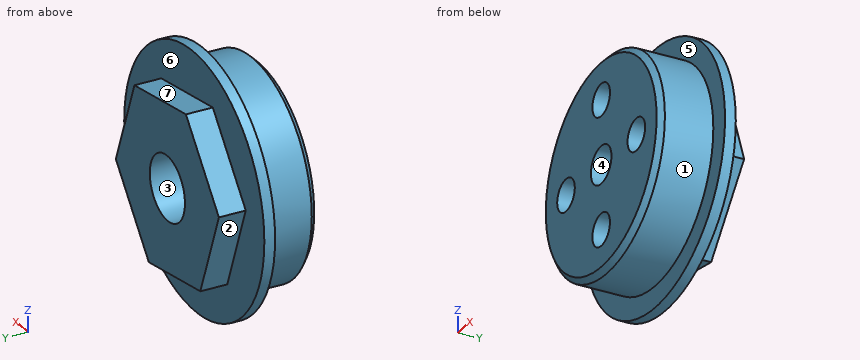
from build123d import *

# Parameters (mm, degrees)
ESQUISSE1_R             = 9.95
BOSS_EXTRU_1_DEPTH      = 6
BOSS_EXTRU_2_DEPTH      = 2.5
ESQUISSE3_R             = 11.95
ESQUISSE3_R_2           = 9.95
BOSS_EXTRU_3_DEPTH      = 1
ESQUISSE4_R             = 1.5
ENL_V_MAT_EXTRU_1_DEPTH = 5
ESQUISSE5_R             = 1.75
ENL_V_MAT_EXTRU_2_DEPTH = 9.5
ESQUISSE6_R             = 3
ENL_V_MAT_EXTRU_3_DEPTH = 3.5
CHANFREIN1_SIZE         = 0.5


with BuildPart() as part:
    # Esquisse1 → Boss.-Extru.1 (new body)
    with BuildSketch(Plane(origin=(0, 0, 0), x_dir=(1, 0, 0), z_dir=(0, 1, 0))):
        Circle(ESQUISSE1_R)
    extrude(amount=BOSS_EXTRU_1_DEPTH)

    # Esquisse2 → Boss.-Extru.2 (add)
    with BuildSketch(Plane(origin=(0, 6, 0), x_dir=(1, 0, 0), z_dir=(0, 1, 0))):
        Polygon((-3.162738548, -8.319079569), (5.623164969, -6.898551713), (8.785903517, 1.420527856), (3.162738548, 8.319079569), (-5.623164969, 6.898551713), (-8.785903517, -1.420527856), align=None)
    extrude(amount=BOSS_EXTRU_2_DEPTH)

    # Esquisse3 → Boss.-Extru.3 (add)
    with BuildSketch(Plane(origin=(0, 6, 0), x_dir=(1, 0, 0), z_dir=(0, 1, 0))):
        Circle(ESQUISSE3_R)
        Circle(ESQUISSE3_R_2, mode=Mode.SUBTRACT)
    extrude(amount=-BOSS_EXTRU_3_DEPTH)

    # Esquisse4 → Enlèv. mat.-Extru.1 (cut)
    with BuildSketch(Plane.XZ):
        with Locations((0, 6)):
            Circle(ESQUISSE4_R)
        with Locations((6, 0)):
            Circle(ESQUISSE4_R)
        with Locations((0, -6)):
            Circle(ESQUISSE4_R)
        with Locations((-6, 0)):
            Circle(ESQUISSE4_R)
    extrude(amount=-ENL_V_MAT_EXTRU_1_DEPTH, mode=Mode.SUBTRACT)

    # Esquisse5 → Enlèv. mat.-Extru.2 (cut, through all)
    with BuildSketch(Plane.XZ):
        Circle(ESQUISSE5_R)
    extrude(amount=-ENL_V_MAT_EXTRU_2_DEPTH, mode=Mode.SUBTRACT)

    # Esquisse6 → Enlèv. mat.-Extru.3 (cut)
    with BuildSketch(Plane(origin=(0, 8.5, 0), x_dir=(1, 0, 0), z_dir=(0, 1, 0))):
        Circle(ESQUISSE6_R)
    extrude(amount=-ENL_V_MAT_EXTRU_3_DEPTH, mode=Mode.SUBTRACT)

    # Chanfrein1
    chanfrein1_edges = [part.edges().sort_by_distance(p)[0] for p in [
        (-9.95, 0, 0),
    ]]
    chamfer(chanfrein1_edges, length=CHANFREIN1_SIZE)


solid = part.part
The model under review builds one solid part; all positions refer to its coordinate system, in mm. Face numbers are marked on the shaded views. A direction names the side the tool comes from. Give positions to 0.01 mm unless a question says otherwise; leave off trailing zeros. Loops run counter-clockwise (first coordinate to the right, second up) from the corner with the lowest first, then second, coordinate; pieces in that order, holes last. Notation, with made-up numbers: (-1, 58) -> (48, 58) arc R9 cw to (48, 64) -> close; hole circle Ø7 at (-40, 54.25). An arc over 180 degrees is marked (long way). Write each question's results on one line, items separated by ' | '.
1) Insertion check: pin 1 Ø4 at (x, y) = (-6.5, 1) entering from -Z; pin 2 Ø1.5 at (y, z) = (5.5, 7.5) entering from +X; pin 3 Ø3 at (y, z) = (2, 7.5) entering from +X. Each pin has a flat end and moves straight along its axis. Give the tip position at first contact, or say it passes through.
Conclusion:
pin 1: stops at z = -8.87 | pin 2: stops at x = 9.86 | pin 3: stops at x = 7.94
2) For line 1 along Z through (x, y) = (0, 3.4); line 2 along X through (y, z) = (2.25, 0.75); line 3 along Y through (x, z) = (6.5, 9.25), list the stretches that pass through material, from the lowest coordinate up. Write a range as from..to.
Conclusion:
line 1: z = -9.95..-7.5, -4.5..-1.75, 1.75..4.5, 7.5..9.95 | line 2: x = -9.92..-7.3, -4.7..-1.58, 1.58..4.7, 7.3..9.92 | line 3: y = 5..6
3) Draft analysis for pull direction X (two halves, no side actions). For the marked faces 1, 2, 3 and 4, state which applies: pulls with the +X half, pulls with the -X half, needs draft (parallel to the pull), parting line crosses it, or undercut.
Conclusion:
face 1: parting line crosses it | face 2: pulls with the -X half | face 3: undercut | face 4: undercut
4) Tool access review of the marked faces 5, 6 and 7: name each direction out of +Z, -Z, +X, -X, +Y, -Y from which nothing blocks a thin tool from reaching the whole face with its end or side.
Conclusion:
face 5: -Y | face 6: +Y | face 7: +Z, +X, +Y
5) Take a section at A-A, the plane y = 4.25. Give the boundary of the cut face in (x, z).
Conclusion:
outline: circle Ø19.9 at (0, 0); hole circle Ø3 at (-6, 0); hole circle Ø3.5 at (0, 0); hole circle Ø3 at (0, -6); hole circle Ø3 at (0, 6); hole circle Ø3 at (6, 0)
